```python
from build123d import *

# Parameters (mm, degrees)
F1_DEPTH      = 25
F0_R          = 16
F2_DEPTH      = 36
F4_DEPTH      = 10
F6_DEPTH      = 10
F8_R          = 19
F8_R_2        = 10
F9_DEPTH      = 8
F10_T4_DEPTH  = 103
F10_S6_R      = 25
F10_T7_DEPTH  = 53
F10_T11_DEPTH = 103
F10_S13_R     = 25
F10_T14_DEPTH = 53


# Not quite as in the source:
# - a fillet or chamfer that OpenCascade refuses, or shapes differently, is made with other operations: its cross-section is extruded or revolved along the edge and cut away or added
# - a pattern or mirror of a feature is missing from the dataset's text; its kind, count and spacing are read off the source's solid


with BuildPart() as f1:
    # F0 (on Top) → F1 (new body)
    with BuildSketch(Plane.XY):
        with BuildLine():
            Line((-35, 44), (-75, 44))
            Line((-75, 44), (-75, 34))
            Line((-75, 34), (-51, 34))
            ThreePointArc((-51, 34), (-46.7573593129, 32.2426406871), (-45, 28))
            Line((-45, 28), (-45, 21))
            ThreePointArc((-45, 21), (-41.4852813742, 12.5147186258), (-33, 9))
            Line((-33, 9), (-25, 9))
            Line((-25, 9), (-25, -16))
            ThreePointArc((-25, -16), (0, 9), (25, -16))
            Line((25, -16), (25, 9))
            Line((25, 9), (33, 9))
            ThreePointArc((33, 9), (41.4852813742, 12.5147186258), (45, 21))
            Line((45, 21), (45, 28))
            ThreePointArc((45, 28), (46.7573593129, 32.2426406871), (51, 34))
            Line((51, 34), (75, 34))
            Line((75, 34), (75, 44))
            Line((75, 44), (35, 44))
            Line((35, 44), (35, 34))
            Line((35, 34), (35, 22))
            ThreePointArc((35, 22), (34.1213203436, 19.8786796564), (32, 19))
            Line((32, 19), (-32, 19))
            ThreePointArc((-32, 19), (-34.1213203436, 19.8786796564), (-35, 22))
            Line((-35, 22), (-35, 34))
            Line((-35, 34), (-35, 44))
        make_face()
    extrude(amount=F1_DEPTH)

    # F0 (on Top) → F2 (join)
    with BuildSketch(Plane.XY):
        with BuildLine():
            ThreePointArc((25, -16), (0, 9), (-25, -16))
            ThreePointArc((-25, -16), (0, -41), (25, -16))
        make_face()
        with Locations((0, -16)):
            Circle(F0_R, mode=Mode.SUBTRACT)
    extrude(amount=F2_DEPTH)

    # F3 (on face) → F4 (join)
    with BuildSketch(Plane.XY):
        with BuildLine():
            Line((75, 34), (75, 44))
            Line((75, 44), (-75, 44))
            Line((-75, 44), (-75, 34))
            ThreePointArc((-75, 34), (-70.7573593129, 32.2426406871), (-69, 28))
            Line((-69, 28), (-69, 8))
            ThreePointArc((-69, 8), (-65.4852813742, -0.4852813742), (-57, -4))
            ThreePointArc((-57, -4), (-48.5147186258, -7.5147186258), (-45, -16))
            Line((-45, -16), (-45, -44))
            Line((-45, -44), (45, -44))
            Line((45, -44), (45, -16))
            ThreePointArc((45, -16), (48.5147186258, -7.5147186258), (57, -4))
            ThreePointArc((57, -4), (65.4852813742, -0.4852813742), (69, 8))
            Line((69, 8), (69, 28))
            ThreePointArc((69, 28), (70.7573593129, 32.2426406871), (75, 34))
        make_face()
    extrude(amount=-F4_DEPTH)

    # F5 (on face) → F6 (join)
    with BuildSketch(Plane.YZ.offset(45)):
        with BuildLine():
            ThreePointArc((-34.7712820587, -68.9392124579), (-17.4740489959, -47.0572657845), (3, -66))
            ThreePointArc((3, -66), (2.6502712249, -69.6286889144), (1.6139596592, -73.1237928888))
            Line((1.6139596592, -73.1237928888), (20.8237372905, -25.6265883042))
            ThreePointArc((20.8237372905, -25.6265883042), (30.0238648475, -14.2715739575), (44, -10))
            Line((44, -10), (34, -10))
            Line((34, -10), (-16, -10))
            Line((-16, -10), (-44, -10))
            Line((-44, -10), (-34.7712820587, -68.9392124579))
        make_face()
    f6 = extrude(amount=-F6_DEPTH)

    # F6_copies: F6 across plane
    add(f6.mirror(Plane(origin=(0, 0, 0), x_dir=(0, 0, -1), z_dir=(-1, 0, 0))))

    # F8 (on face) → F9 (join, symmetric)
    with BuildSketch(Plane.YZ.offset(40)):
        with Locations((-16, -66)):
            Circle(F8_R)
        with Locations((-16, -66)):
            Circle(F8_R_2, mode=Mode.SUBTRACT)
    f9 = extrude(amount=F9_DEPTH, both=True)

    # F9_copies: F9 across plane
    add(f9.mirror(Plane(origin=(0, 0, 0), x_dir=(0, 0, -1), z_dir=(-1, 0, 0))))

    # F10: fillet of radius 6 on 2 edges, made by hand


with BuildPart() as f10_tool2:
    # F10_s3 → F10_t4 (new body)
    with BuildSketch(Plane.XZ.offset(-44)):
        with BuildLine():
            ThreePointArc((29, -10), (33.2426406871, -11.7573593129), (35, -16))
            Line((35, -16), (35, -10))
            Line((35, -10), (29, -10))
        make_face()
    extrude(amount=F10_T4_DEPTH)

    split(bisect_by=Plane(origin=(0, -44.4753827877, -6.9639675517), x_dir=(1, 0, 0), z_dir=(0, 0.9879622136, 0.1546953925)), keep=Keep.TOP)

    # F10_s6 → F10_t7 (cut, symmetric)
    with BuildSketch(Plane.YZ.offset(32)):
        with Locations((44, -35)):
            Circle(F10_S6_R)
    extrude(amount=F10_T7_DEPTH, both=True, mode=Mode.SUBTRACT)


with BuildPart() as f1_1:
    add(f1.part)

    # F10_t1: union F10_tool2
    add(f10_tool2.part)


with BuildPart() as f10_tool9:
    # F10_s10 → F10_t11 (new body)
    with BuildSketch(Plane.XZ.offset(-44)):
        with BuildLine():
            ThreePointArc((-35, -16), (-33.2426406871, -11.7573593129), (-29, -10))
            Line((-29, -10), (-35, -10))
            Line((-35, -10), (-35, -16))
        make_face()
    extrude(amount=F10_T11_DEPTH)

    split(bisect_by=Plane(origin=(0, -44.4753827877, -6.9639675517), x_dir=(1, 0, 0), z_dir=(0, 0.9879622136, 0.1546953925)), keep=Keep.TOP)

    # F10_s13 → F10_t14 (cut, symmetric)
    with BuildSketch(Plane.YZ.offset(-32)):
        with Locations((44, -35)):
            Circle(F10_S13_R)
    extrude(amount=F10_T14_DEPTH, both=True, mode=Mode.SUBTRACT)


with BuildPart() as f1_2:
    add(f1_1.part)

    # F10_t8: union F10_tool9
    add(f10_tool9.part)


solid = f1_2.part
```
Geometry: final body of the model. Coordinates: model frame, mm. A direction names the side the tool comes from. Round coordinates to 2 decimals unless told otherwise and drop trailing zeros. Loops run counter-clockwise (first coordinate to the right, second up) from the corner with the lowest first, then second, coordinate; pieces in that order, holes last. Notation, with made-up numbers: (54, -27.5) -> (63, -27.5) arc R17 cw to (63, -13.5) -> close; hole circle Ø7 at (31, 39.25). An arc over 180 degrees is marked (long way). Use one line per item in the form item = value.
Item 1: Access query for faces 5 (the flat face through (0, 19, 12)), 6 (the flat face through (45, 24, 12)), 7 (the flat face through (32, -8, -74)). Directions: +Z, -Z, +X, -X, +Y, -Y. A direction counts if a zero-diameter tool reaches every point of the face in a straight line with its end or side. Return the directions, or none.
Evaluation:
face_5 = +Z, +Y
face_6 = +Z, +X, -Y
face_7 = -Z, +Y, -Y
Item 2: Cut plane C-C on z = -4. Output: boundary loops of the cut face in (x, y), then the cut area to 3 significant figures.
Evaluation:
outline = (-75, 34) arc R6 cw to (-69, 28) -> (-69, 8) arc R12 ccw to (-57, -4) arc R12 cw to (-45, -16) -> (-45, -44) -> (45, -44) -> (45, -16) arc R12 cw to (57, -4) arc R12 ccw to (69, 8) -> (69, 28) arc R6 cw to (75, 34) -> (75, 44) -> (-75, 44) -> close
area = 10,400 mm2
Item 3: Cut plane B-B on x = -37. Output: boundary loops of the cut face in (y, z).
Evaluation:
outline = (-44, -10) -> (-34.77, -68.94) arc R19 ccw to (1.61, -73.12) -> (20.82, -25.63) arc R25 cw to (44, -10) -> (44, 25) -> (9.69, 25) -> (9.69, 0) -> (-44, 0) -> close; hole circle Ø20 at (-16, -66)
Item 4: Contact query for flat-ended pins moving along their axis: pin 1 Ø12 at (x, z) = (-58.5, 8) entering from -Y; pin 2 Ø2 at (x, y) = (-28.5, 31.5) entering from -Z; pin 3 Ø22 at (y, z) = (-20, -40.5) entering from -X. Output: stop coordinate, or through.
Evaluation:
pin_1 = 34
pin_2 = -10.02
pin_3 = -48
Item 5: Draft query along Z for faces 1 (the flat face through (0, 1, -10)), 2 (the flat face through (-34, -4, 0)), 3 (the flat face through (63, 34, 12)), 4 (the cylindrical face through (-39.888, -6.763, -69.83)). Return one class per face: released by +Z, released by -Z, zero draft, split by the parting line, or undercut.
Evaluation:
face_1 = released by -Z
face_2 = released by +Z
face_3 = zero draft
face_4 = undercut
Item 6: Material intervals for probe 1 along Z at (x, y) = (40, -16); probe 2 along X at (y, z) = (-37, -30); probe 3 along Z at (x, y) = (32.5, -25), sorted ascending.
Evaluation:
probe_1 = -85 to -76, -56 to 0
probe_2 = -45 to -35, 35 to 45
probe_3 = -82.73 to -70.36, -61.64 to -49.27, -11.13 to 0
Item 7: Cut plane D-D on y = -18.5. Give the number of separate pieces and of enclosed holes in the cut face, then the cut area to 3 significant figures.
Evaluation:
separate_pieces = 3
enclosed_holes = 0
area = 2,900 mm2
Item 8: Cut plane A-A on z = -52. Output: boundary loops of the cut face in (x, y), then the cut area to 3 significant figures.
Evaluation:
outline = (-48, -28.85) -> (-45, -28.85) -> (-45, -37.42) -> (-35, -37.42) -> (-35, -28.85) -> (-32, -28.85) -> (-32, -3.15) -> (-35, -3.15) -> (-35, 10.16) -> (-45, 10.16) -> (-45, -3.15) -> (-48, -3.15) -> close; (32, -28.85) -> (35, -28.85) -> (35, -37.42) -> (45, -37.42) -> (45, -28.85) -> (48, -28.85) -> (48, -3.15) -> (45, -3.15) -> (45, 10.16) -> (35, 10.16) -> (35, -3.15) -> (32, -3.15) -> close
area = 1,260 mm2
